from build123d import *

# Parameters (mm, degrees)
F1_DEPTH  = 16
F2_W      = 70
F2_H      = 3
F3_DEPTH  = 2
F4_W      = 50
F4_H      = 14
F5_DEPTH  = 2
F6_R      = 1
F9_DEPTH  = 2
F11_DEPTH = 42.001
F13_D     = 4
F14_R     = 3
F14_R_2   = 2
F15_DEPTH = 5
F16_R     = 3


# Not quite as in the source:
# - a pattern or mirror of a feature is missing from the dataset's text; its kind, count and spacing are read off the source's solid


with BuildPart() as f1:
    # F0 (on Front) → F1 (new body)
    with BuildSketch(Plane.XZ):
        with BuildLine():
            ThreePointArc((0, -9), (-9, 0), (0, 9))
            Line((0, 9), (94, 9))
            Line((94, 9), (94, 11))
            Line((94, 11), (0, 11))
            ThreePointArc((0, 11), (-11, 0), (0, -11))
            Line((0, -11), (19, -11))
            ThreePointArc((19, -11), (21.7681124643, -11.8361612201), (23.6103896104, -14.064978646))
            ThreePointArc((23.6103896104, -14.064978646), (52.5045279084, -47.666837229), (95.6038093767, -57.9822657286))
            ThreePointArc((95.6038093767, -57.9822657286), (102.8775016632, -58.177663117), (109.0707194958, -61.9971961375))
            Line((109.0707194958, -61.9971961375), (110.8678187413, -61))
            ThreePointArc((110.8678187413, -61), (103.7692922231, -56.3602117831), (95.2965735981, -56))
            ThreePointArc((95.2965735981, -56), (52.955209083, -45.5949761441), (24.9861322889, -12.1467114099))
            ThreePointArc((24.9861322889, -12.1467114099), (23.1470623984, -9.8607704249), (20.3422845953, -9))
            Line((20.3422845953, -9), (0, -9))
        make_face()
    extrude(amount=F1_DEPTH)

    # F2 (on face) → F3 (join)
    with BuildSketch(Plane.XY.offset(11)):
        with Locations((59, -17.5)):
            Rectangle(F2_W, F2_H)
    extrude(amount=-F3_DEPTH)

    # F4 (on face) → F5 (join)
    with BuildSketch(Plane.XZ.offset(19)):
        with Locations((69, 4)):
            Rectangle(F4_W, F4_H)
    extrude(amount=F5_DEPTH)

    # F6
    f6_edges = [f1.edges().sort_by_distance(p)[0] for p in [
        (69, -21, 11),
        (34, -19, 11),
    ]]
    fillet(f6_edges, radius=F6_R)

    # F7: F1 across plane


with BuildPart() as f1_1:
    add(f1.part)
    add(f1.part.mirror(Plane.XZ))

    # F8 (on face) → F9 (cut)
    with BuildSketch(Plane.XY.offset(11)):
        with BuildLine():
            Line((94, 12), (34, 12))
            ThreePointArc((34, 12), (22, 0), (34, -12))
            Line((34, -12), (94, -12))
            Line((94, -12), (94, 12))
        make_face()
    extrude(amount=-F9_DEPTH, mode=Mode.SUBTRACT)

    # F10 (on face) → F11 (cut, through all)
    with BuildSketch(Plane.XZ.offset(21)):
        with BuildLine():
            ThreePointArc((50, 5), (47, 2), (50, -1))
            Line((50, -1), (70, -1))
            ThreePointArc((70, -1), (73, 2), (70, 5))
            Line((70, 5), (50, 5))
        make_face()
    extrude(amount=-F11_DEPTH, mode=Mode.SUBTRACT)

    # F13 (through all)
    with Locations(Plane.XZ.offset(21)):
        with Locations((80, 3)):
            Hole(F13_D / 2)

    # F14 (on face) → F15 (join)
    with BuildSketch(Plane(origin=(0, -19, 0), x_dir=(-1, 0, 0), z_dir=(0, 1, 0))):
        with Locations((-80, 3)):
            Circle(F14_R)
        with Locations((-80, 3)):
            Circle(F14_R_2, mode=Mode.SUBTRACT)
    f15 = extrude(amount=F15_DEPTH)

    # F15_copies: F15 across plane
    add(f15.mirror(Plane.ZX))

    # F16
    f16_edges = [f1_1.edges().sort_by_distance(p)[0] for p in [
        (44, -20, -3),
        (94, -20, -3),
        (94, 20, -3),
        (44, 20, -3),
    ]]
    fillet(f16_edges, radius=F16_R)


solid = f1_1.part
Part model, mm, in its own coordinate system. A direction names the side the tool comes from. Give positions to 0.01 mm unless a question says otherwise; leave off trailing zeros. Loops run counter-clockwise (first coordinate to the right, second up) from the corner with the lowest first, then second, coordinate; pieces in that order, holes last. Notation, with made-up numbers: M 86,23 L 137,23 A10 ccw 137,37 Z; hole C -7.5,35 d11. An arc over 180 degrees is marked long. Put each result on its own line as item: value. Start each with the question number.
1) Saw through at C-C (x = 80). State how many separate pieces and enclosed holes the cut face has, then the cut area to 3 significant figures.
2) Saw through at A-A (x = 10). List the corners of the cut face in (y, z), then the cut area to 3 significant figures.
3) Saw through at B-B (x = 37). List the corners of the cut face in (y, z).
4) Probe probe 1 along Z at (x, y) = (80, -16.65); probe 2 along Z at (x, y) = (1.5, 8.5); probe 3 along Y at (x, z) = (82, 0.5). List the from-to ranges inside material, lowest first.
5) Pull direction Z, two halves, no side cores. Call faces 1 (the cylindrical face through (83, 17, 3)), 2 (the flat face through (36, 13, 11)), 3 (the cylindrical face through (44.9, -20.01, -2.14)): +Z half, -Z half, draft (parallel to the pull), parting line (faces both ways), or undercut.
6) Saw through at D-D (y = -4.5). List the corners of the cut face in (x, z).
7) 3-axis set-ups, long thin cutter, end or side, ignore diameter. For faces 4 (the flat face through (9, 0, -11)), 5 (the flat face through (31.6, 16, -25.3)), 6 (the flat face through (36, -13, 9)), 7 (the cylindrical face through (22, 0, 10)): which of +Z, -Z, +X, -X, +Y, -Y reach the whole face in a straight line?
8) Flat gauge pins, fed straight in: pin 1 (1.1 mm diameter, centred on x = 32.5, z = 9.5, fed in from -Y); pin 2 (21 mm diameter, centred on x = 11, y = 3.5, fed in from -Z); pin 3 (1 mm diameter, centred on x = 85, y = -2, fed in from -Z); pin 4 (10 mm diameter, centred on x = 84, y = 11.5, fed in from +Z). Where does each tip first touch, or does it go through?
Numbers:
1. separate pieces: 5
1. enclosed holes: 0
1. area: 152 mm^2
2. outline: M -16,-11 L 16,-11 L 16,-9 L -16,-9 Z; M -16,9 L 16,9 L 16,11 L -16,11 Z
2. area: 128 mm^2
3. outline: M -19,9 L -12,9 L -12,11 L -18,11 A1 ccw -19,10 Z; M -16,-34.93 L 16,-34.93 L 16,-31.93 L -16,-31.93 Z; M 12,9 L 19,9 L 19,10 A1 ccw 18,11 L 12,11 Z
4. probe 1: 0 to 1, 5 to 6, 9 to 11
4. probe 2: -11 to -9, 9 to 11
4. probe 3: -21 to -19, 19 to 21
5. face 1: undercut
5. face 2: +Z half
5. face 3: -Z half
6. outline: M 0,-11 L 19,-11 A5 cw 23.61,-14.06 A72 ccw 95.6,-57.98 A14 cw 109.07,-62 L 110.87,-61 A16 ccw 95.3,-56 A70 cw 24.99,-12.15 A5 ccw 20.34,-9 L 0,-9 A9 cw 0,9 L 22.88,9 L 22.88,11 L 0,11 A11 ccw Z
7. face 4: -Z, -X, +Y, -Y
7. face 5: -Z, -X, +Y
7. face 6: +X
7. face 7: +Z, +X
8. pin 1: y = -19
8. pin 2: z = -11.67
8. pin 3: z = -58.06
8. pin 4: z = 11
